Autodesk Inventor part; units mm, degrees
ref_plane "YZ Plane" through (0, 0, 0) normal (1, 0, 0) x (0, 1, 0)
ref_plane "XZ Plane" through (0, 0, 0) normal (0, 1, 0) x (-1, 0, 0)
ref_plane "XY Plane" through (0, 0, 0) normal (0, 0, 1) x (1, 0, 0)
sketch "Sketch1" plane through (0, 0, 0) normal (0, 0, 1) x (1, 0, 0)
  circle A0 centre (0, 0) radius 6.35
  circle A1 centre (0, 0) radius 3
  dimension "d0" = 12.7
  dimension "d1" = 6
extrude "Extrusion1" add sketch "Sketch1" along normal blind 150 contours A0 | A1
sketch "Sketch2" plane through (0, 0, 150) normal (0, 0, 1) x (1, 0, 0)
  circle A0 centre (0, 0) radius 3
  dimension "d4" = 6
extrude "Extrusion2" cut sketch "Sketch2" against normal blind 25
extrude "Extrusion3" cut sketch "Sketch1" along normal blind 25 contours A1
thread "Thread1"
thread "Thread2"
sketch "Boceto3" plane through (0, 0, 150) normal (0, 0, 1) x (1, 0, 0)
  circle A0 centre (0, 0) radius 7
  circle A1 centre (0, 0) radius 4
  dimension "d13" = 8
  dimension "d20" = 14
sketch "Boceto4" plane through (0, 0, 0) normal (0, 0, -1) x (-1, 0, 0)
  circle A0 centre (0, 0) radius 7
  circle A1 centre (0, 0) radius 4
  dimension "d14" = 8
  dimension "d19" = 14
extrude "Extrusión4" cut sketch "Boceto4" against normal blind 10
extrude "Extrusión5" cut sketch "Boceto3" against normal blind 10
properties part number "Guías de Soporte de Motor" material "Steel, High Strength, Low Alloy"
Input: part model. Units: mm. Frame: model coordinates. A direction names the side the tool comes from. Give positions to 0.01 mm unless a question says otherwise; leave off trailing zeros. Write each loop counter-clockwise with the first axis right and the second up, starting at its lowest first coordinate (ties: lowest second). Pieces come first, ordered by that corner, then holes. Notation, with made-up numbers: (-6.75, 29.5) - (51.25, 29.5) arc R8 cw to (51.25, 37.5) - close; hole circle Ø11 at (-26.75, -33.75). An arc over 180 degrees is marked (long way). Write item = value, one per line. Start each with the question number.
1. Section query C-C, the plane z = 115.5. Output: boundary loops of the cut face in (x, y), then the cut area to 3 significant figures.
2. Ray query, L1, parallel to Y at x = 0, z = 10.25; L2, parallel to Y at x = 0, z = 9; L3, parallel to Z at x = -2, y = -2. Return the intervals inside material, ascending.
3. Access query for faces 4 (the flat face through (0, 0, 125)), 5 (the flat face through (0, 0, 25)), 6 (the flat face through (1, 3, 150)). Directions: +Z, -Z, +X, -X, +Y, -Y. A direction counts if a zero-diameter tool reaches every point of the face in a straight line with its end or side. Return the directions, or none.
4. First-contact query: pin 1 Ø1.8 at (x, y) = (0, -0.5) entering from -Z; pin 2 Ø6.5 at (x, y) = (2.5, 1.5) entering from -Z; pin 3 Ø1 at (x, y) = (3, 3.5) entering from -Z; pin 4 Ø1.5 at (x, z) = (-4.5, 62.5) entering from -Y. Flat tips, straight axial feed; report the tip coordinate or a pass-through.
5. Section query A-A, the plane x = 0. Output: boundary loops of the cut face in (y, z).
6. Mould query, pull axis Y, two halves, no side actions, for faces 1 (the flat face through (1, 3, 0)), 2 (the cylindrical face through (-3, 0, 138)), 3 (the cylindrical face through (-1.38, 6.2, 74.09)). Classes: released by +Y, released by -Y, zero draft, split by the parting line, or undercut.
Check sheet entries:
q1.outline = circle Ø12.7 at (0, 0)
q1.area = 127 mm2
q2.L1 = -6.35 to -3, 3 to 6.35
q2.L2 = -4 to -3, 3 to 4
q2.L3 = 25 to 125
q3.face_4 = +Z
q3.face_5 = -Z
q3.face_6 = +Z, +X, -X, +Y, -Y
q4.pin_1 = 25
q4.pin_2 = 0
q4.pin_3 = 10
q4.pin_4 = -5.12
q5.outline = (-6.35, 10) - (-4, 10) - (-4, 0) - (-3, 0) - (-3, 25) - (3, 25) - (3, 0) - (4, 0) - (4, 10) - (6.35, 10) - (6.35, 140) - (4, 140) - (4, 150) - (3, 150) - (3, 125) - (-3, 125) - (-3, 150) - (-4, 150) - (-4, 140) - (-6.35, 140) - close
q6.face_1 = zero draft
q6.face_2 = undercut
q6.face_3 = split by the parting line
